Model file for the job. Use its own axes, mm. Face numbers are marked on the shaded views. Give positions to 0.01 mm unless a question says otherwise; leave off trailing zeros. Order: outer loops, then holes, each group sorted by start corner. A loop starts at its lowest first (then second) coordinate and runs counter-clockwise, first axis right, second up. Notation, with made-up numbers: (20.25, 49.25) - (64.25, 49.25) arc R4 cw to (64.25, 53.25) - close; hole circle Ø3 at (3, -32.75). An arc over 180 degrees is marked (long way). Use CSV: the item, a comma, the result in double quotes. Start each with the question number.
(1) Band-saw the part on B-B, the plane y = -8.5. Give the cut face in (x, z) (3 decimals).
(2) Probe L1, parallel to X at y = 123, z = 0.25; L2, parallel to Y at x = 32, z = 1.65 (3 decimals); L3, parallel to X at y = -38, z = 1.3. List the from-to ranges inside material, lowest first.
(3) Pull direction Z, two halves, no side cores. Call the marked faces 1 and 2: +Z half, -Z half, draft (parallel to the pull), parting line (faces both ways), or undercut.
(4) Band-saw the part on A-A, the plane x = 28. Give the cut face in (y, z) (3 decimals).
(5) Band-saw the part on C-C, the plane y = 114.5. Give the cut face in (x, z) (3 decimals).
(6) Drop flat-ended pins along their axis: pin 1 Ø1 at (y, z) = (26, 1) entering from -X; pin 2 Ø1 at (x, y) = (21.5, 75.5) entering from -Z; pin 3 Ø0.8 at (y, z) = (34.5, 1.5) entering from +X; pin 4 Ø1.6 at (x, z) = (78.5, 1) entering from +Y. Give the stop position or say it passes through.
from build123d import *

# Parameters (mm, degrees)
SKETCH1_W           = 76.2
SKETCH1_H           = 152.4
BOSS_EXTRUDE1_DEPTH = 3.175
SKETCH2_W           = 3.175
SKETCH2_H           = 12.7
BOSS_EXTRUDE3_DEPTH = 3.175
SKETCH4_W           = 8.89
SKETCH4_H           = 3.302
SKETCH4_W_2         = 2.5
SKETCH4_H_2         = 6.5
CUT_EXTRUDE4_DEPTH  = 3.175
SKETCH5_W           = 76.2
SKETCH5_H           = 44.45
SKETCH5_W_2         = 43
SKETCH5_H_2         = 43
BOSS_EXTRUDE4_DEPTH = 3.175
SKETCH7_W           = 76.2
SKETCH7_H           = 3.81
BOSS_EXTRUDE5_DEPTH = 3.175
FILLET1_R           = 2.54
FILLET2_R           = 1.27


with BuildPart() as part:
    # Sketch1 → Boss-Extrude1 (new body)
    with BuildSketch(Plane.XY):
        with Locations((38.1, 76.2)):
            Rectangle(SKETCH1_W, SKETCH1_H)
    extrude(amount=BOSS_EXTRUDE1_DEPTH)

    # Sketch2 → Boss-Extrude3 (add)
    with BuildSketch(Plane.XY.offset(3.175)):
        with Locations((-1.5875, 76.2)):
            Rectangle(SKETCH2_W, SKETCH2_H)
        with Locations((77.7875, 139.7)):
            Rectangle(SKETCH2_W, SKETCH2_H)
        with Locations((77.7875, 76.2)):
            Rectangle(SKETCH2_W, SKETCH2_H)
        with Locations((77.7875, 12.7)):
            Rectangle(SKETCH2_W, SKETCH2_H)
        with Locations((-1.5875, 12.7)):
            Rectangle(SKETCH2_W, SKETCH2_H)
        with Locations((-1.5875, 139.7)):
            Rectangle(SKETCH2_W, SKETCH2_H)
    extrude(amount=-BOSS_EXTRUDE3_DEPTH)

    # Sketch4 → Cut-Extrude4 (cut)
    with BuildSketch(Plane.XY.offset(3.175)):
        with Locations((4.445, 120.65)):
            Rectangle(SKETCH4_W, SKETCH4_H)
        with Locations((6.37, 120.65)):
            Rectangle(SKETCH4_W_2, SKETCH4_H_2)
        with Locations((6.37, 31.75)):
            Rectangle(SKETCH4_W_2, SKETCH4_H_2)
        with Locations((4.445, 31.75)):
            Rectangle(SKETCH4_W, SKETCH4_H)
        with Locations((71.755, 31.75)):
            Rectangle(SKETCH4_W, SKETCH4_H)
        with Locations((69.83, 31.75)):
            Rectangle(SKETCH4_W_2, SKETCH4_H_2)
        with Locations((69.83, 120.65)):
            Rectangle(SKETCH4_W_2, SKETCH4_H_2)
        with Locations((71.755, 120.65)):
            Rectangle(SKETCH4_W, SKETCH4_H)
    extrude(amount=-CUT_EXTRUDE4_DEPTH, mode=Mode.SUBTRACT)

    # Sketch5 → Boss-Extrude4 (add)
    with BuildSketch(Plane.XY.offset(3.175)):
        with Locations((38.1, -22.225)):
            Rectangle(SKETCH5_W, SKETCH5_H)
        with Locations((38.1, -22.225)):
            Rectangle(SKETCH5_W_2, SKETCH5_H_2, mode=Mode.SUBTRACT)
    extrude(amount=-BOSS_EXTRUDE4_DEPTH)

    # Sketch7 → Boss-Extrude5 (add)
    with BuildSketch(Plane.XY.offset(3.175)):
        with Locations((38.1, -46.355)):
            Rectangle(SKETCH7_W, SKETCH7_H)
    extrude(amount=-BOSS_EXTRUDE5_DEPTH)

    # Fillet1
    fillet1_edges = [part.edges().sort_by_distance(p)[0] for p in [
        (76.2, -48.26, 1.5875),
        (0, -48.26, 1.5875),
    ]]
    fillet(fillet1_edges, radius=FILLET1_R)

    # Fillet2
    fillet2_edges = [part.edges().sort_by_distance(p)[0] for p in [
        (59.6, -43.725, 1.5875),
        (16.6, -43.725, 1.5875),
        (16.6, -0.725, 1.5875),
        (59.6, -0.725, 1.5875),
    ]]
    fillet(fillet2_edges, radius=FILLET2_R)


solid = part.part
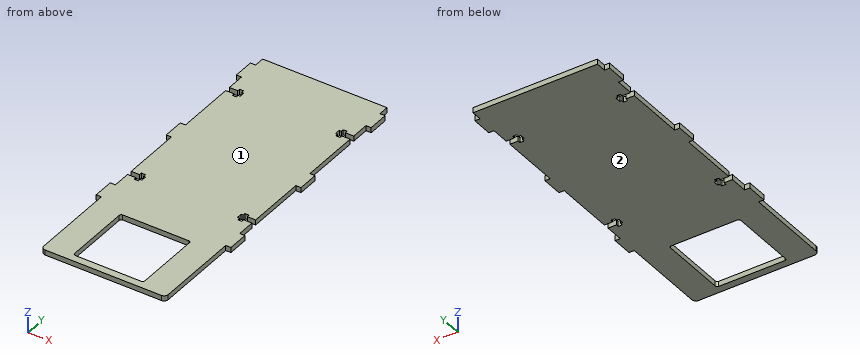
Answer block:
1,outline,"(0, 0) - (16.6, 0) - (16.6, 3.175) - (0, 3.175) - close; (59.6, 0) - (76.2, 0) - (76.2, 3.175) - (59.6, 3.175) - close"
2,L1,"x = 0 to 5.12, 7.62 to 68.58, 71.08 to 76.2"
2,L2,"y = -48.26 to -43.725, -0.725 to 152.4"
2,L3,"x = 0 to 16.6, 59.6 to 76.2"
3,face 1,"+Z half"
3,face 2,"-Z half"
4,outline,"(-48.26, 0) - (-43.725, 0) - (-43.725, 3.175) - (-48.26, 3.175) - close; (-0.725, 0) - (152.4, 0) - (152.4, 3.175) - (-0.725, 3.175) - close"
5,outline,"(0, 0) - (76.2, 0) - (76.2, 3.175) - (0, 3.175) - close"
6,pin 1,"stops at x = 0"
6,pin 2,"stops at z = 0"
6,pin 3,"stops at x = 76.2"
6,pin 4,"stops at y = 146.05"
